Source: CAD feature listing. Evaluate the final solid. Frame: model axes, mm. A direction names the side the tool comes from. Coordinates: 2 decimals unless noted, no trailing zeros. Order: outer loops, then holes, each group sorted by start corner. A loop starts at its lowest first (then second) coordinate and runs counter-clockwise, first axis right, second up. Notation, with made-up numbers: (21.25, 18.25) -> (48.25, 18.25) arc R18 cw to (48.25, 47.25) -> close; hole circle Ø11 at (-20, 5.25). An arc over 180 degrees is marked (long way). Put each result on its own line as item: value.
from build123d import *

# Parameters (mm, degrees)
SKETCH1_W            = 10
SKETCH1_H            = 10
BOSS_EXTRUDE1_DEPTH  = 2
FILLET2_R            = 1
FILLET3_R            = 1
FILLET5_R            = 0.5
SKETCH6_W            = 8
SKETCH6_H            = 8
BOSS_EXTRUDE2_DEPTH  = 20
FILLET7_R            = 1
M3_CLEARANCE_HOLE1_D = 3.4
CUT_EXTRUDE1_DEPTH   = 20


with BuildPart() as part:
    # Sketch1 → Boss-Extrude1 (new body)
    with BuildSketch(Plane.XY):
        with Locations((-9.082568807, 1.399082569)):
            Rectangle(SKETCH1_W, SKETCH1_H)
    extrude(amount=BOSS_EXTRUDE1_DEPTH)

    # Fillet2
    fillet2_edges = [part.edges().sort_by_distance(p)[0] for p in [
        (-14.082568807, 6.399082569, 1),
        (-4.082568807, 6.399082569, 1),
        (-14.082568807, -3.600917431, 1),
    ]]
    fillet(fillet2_edges, radius=FILLET2_R)

    # Fillet3
    fillet3_edges = [part.edges().sort_by_distance(p)[0] for p in [
        (-4.082568807, -3.600917431, 1),
    ]]
    fillet(fillet3_edges, radius=FILLET3_R)

    # Fillet5
    fillet5_edges = [part.edges().sort_by_distance(p)[0] for p in [
        (-9.082568807, 6.399082569, 0),
        (-14.082568807, 1.399082569, 0),
        (-9.082568807, -3.600917431, 0),
        (-13.789675589, -3.308024212, 0),
        (-13.789675589, 6.10618935, 0),
        (-4.375462026, 6.10618935, 0),
        (-4.082568807, 1.399082569, 0),
        (-4.375462026, -3.308024212, 0),
    ]]
    fillet(fillet5_edges, radius=FILLET5_R)

    # Sketch6 → Boss-Extrude2 (add)
    with BuildSketch(Plane.XY.offset(2)):
        with Locations((-9.082568807, 1.399082569)):
            Rectangle(SKETCH6_W, SKETCH6_H)
    extrude(amount=BOSS_EXTRUDE2_DEPTH)

    # Fillet7
    fillet7_edges = [part.edges().sort_by_distance(p)[0] for p in [
        (-13.082568807, 5.399082569, 12),
        (-13.082568807, -2.600917431, 12),
        (-5.082568807, -2.600917431, 12),
        (-5.082568807, 5.399082569, 12),
    ]]
    fillet(fillet7_edges, radius=FILLET7_R)

    # M3 Clearance Hole1 (through all)
    with Locations(Plane(origin=(0, 0, 0), x_dir=(-1, 0, 0), z_dir=(0, 0, -1))):
        with Locations((9.082568807, 1.399082569)):
            Hole(M3_CLEARANCE_HOLE1_D / 2)

    # Sketch7 → Cut-Extrude1 (cut)
    with BuildSketch(Plane.XY.offset(22)):
        Polygon((-6.633079065, -1.050407174), (-5.736503592, 2.295658041), (-8.185993335, 4.745147784), (-11.53205855, 3.848572312), (-12.428634022, 0.502507097), (-9.97914428, -1.946982646), align=None)
    extrude(amount=-CUT_EXTRUDE1_DEPTH, mode=Mode.SUBTRACT)


solid = part.part
1. Set-up query: faces 1 (the flat face through (-9, 5.399, 12)), 2 (the flat face through (-13.6, 1.5, 2)), 3 (the flat face through (-9, 6.399, 1)), 4 (the cylindrical face through (-13, -2, 12)). Return all of +Z, -Z, +X, -X, +Y, -Y with unobstructed straight access to the full face (end or side cutting, diameter ignored); none if empty.
Numbers:
face 1: +Z, +X, -X, +Y
face 2: +Z
face 3: +Z, -Z, +X, -X, +Y
face 4: +Z, -X, -Y
2. First-contact query: pin 1 (3 mm diameter, centred on y = 4, z = 6, fed in from +X); pin 2 (5.5 mm diameter, centred on x = -9.08, y = 1.4, fed in from +Z); pin 3 (4 mm diameter, centred on x = -10.5, z = 19, fed in from -Y); pin 4 (5.5 mm diameter, centred on x = -9.5, y = 0, fed in from +Z). Flat tips, straight axial feed; report the tip coordinate or a pass-through.
Numbers:
pin 1: stops at x = -5.08
pin 2: stops at z = 2
pin 3: stops at y = -2.6
pin 4: stops at z = 22
3. Pull-direction query (X, two-part tool) for faces 5 (the flat face through (-5.083, 1, 12)), 6 (the flat face through (-13.083, 1, 12)), 7 (the flat face through (-6.94, 3.5, 12.14)); classes: pulls with the +X half, pulls with the -X half, needs draft (parallel to the pull), parting line crosses it, or undercut.
Numbers:
face 5: pulls with the +X half
face 6: pulls with the -X half
face 7: undercut
4. Ray query, line 1 along Z through (x, y) = (-9.75, 5.5); line 2 along Y through (x, z) = (-8.25, 4.5); line 3 along Y through (x, z) = (-6.75, 19.75). Return the intervals inside material, ascending.
Numbers:
line 1: z = 0 to 2
line 2: y = -2.6 to -1.48, 4.73 to 5.4
line 3: y = -2.6 to -1.08, 3.31 to 5.4
5. Cut plane A-A on z = 13.75. Output: boundary loops of the cut face in (x, y), plus the area to 3 significant figures.
Numbers:
outline: (-13.08, -1.6) arc R1 ccw to (-12.08, -2.6) -> (-6.08, -2.6) arc R1 ccw to (-5.08, -1.6) -> (-5.08, 4.4) arc R1 ccw to (-6.08, 5.4) -> (-12.08, 5.4) arc R1 ccw to (-13.08, 4.4) -> close; hole (-12.43, 0.5) -> (-9.98, -1.95) -> (-6.63, -1.05) -> (-5.74, 2.3) -> (-8.19, 4.75) -> (-11.53, 3.85) -> close
area: 32.0 mm2
6. Cut plane B-B on y = 1.75. Output: boundary loops of the cut face in (x, z).
Numbers:
outline: (-14.08, 0.5) arc R0.5 ccw to (-13.58, 0) -> (-10.75, 0) -> (-10.75, 2) -> (-12.09, 2) -> (-12.09, 22) -> (-13.08, 22) -> (-13.08, 2) -> (-14.08, 2) -> close; (-7.42, 0) -> (-4.58, 0) arc R0.5 ccw to (-4.08, 0.5) -> (-4.08, 2) -> (-5.08, 2) -> (-5.08, 22) -> (-5.88, 22) -> (-5.88, 2) -> (-7.42, 2) -> close
